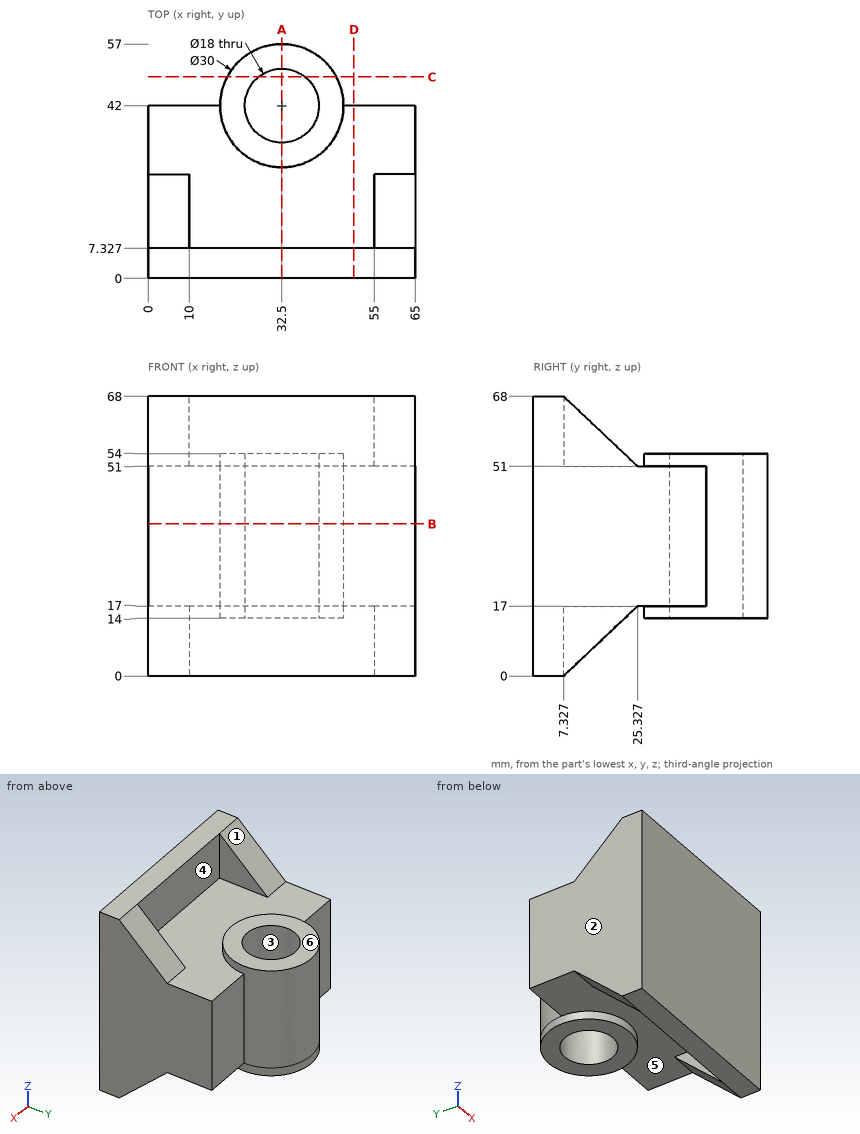
Job drawing, mm, ordinate dimensions from the low corner. One solid piece. A direction names the side the tool comes from. Round coordinates to 2 decimals unless told otherwise and drop trailing zeros. Order: outer loops, then holes, each group sorted by start corner. A loop starts at its lowest first (then second) coordinate and runs counter-clockwise, first axis right, second up. Notation, with made-up numbers: (79, 6) -> (98, 6) arc R21 cw to (98, 31) -> close; hole circle Ø9 at (23.5, 74.5). An arc over 180 degrees is marked (long way). Answer in a Markdown table with one row per item.
1) Mould opens along X. For the marked faces 1, 2 and 3 say: released by +X, released by -X, zero draft, split by the parting line, or undercut.
Values:
| item | result |
|---|---|
| face 1 | zero draft |
| face 2 | released by -X |
| face 3 | undercut |
2) Band-saw the part on B-B on z = 37. Give the cut face in (x, y), and give its area (3 significant figures).
Values:
| item | result |
|---|---|
| outline | (0, 0) -> (65, 0) -> (65, 42) -> (47.5, 42) arc R15 ccw to (17.5, 42) -> (0, 42) -> close; hole circle Ø18 at (32.5, 42) |
| area | 2,830 mm2 |
3) Wall check: L1, parallel to Y at x = 32, z = 28; L2, parallel to Y at x = 25, z = 53 (1 decimal); L3, parallel to Z at x = 13.5, y = 25. Give the ranges that are in metal, low to high.
Values:
| item | result |
|---|---|
| L1 | 0 to 33.01, 50.99 to 56.99 |
| L2 | 0 to 7.3, 29 to 37, 47 to 55 |
| L3 | 17 to 51 |
4) Pin check, flat tips, straight feed: P1, Ø13.5, axis at x = 33, z = 9.5, coming from the +Y side; P2, Ø14.5, axis at x = 32.5, y = 42, coming from the -Z side; P3, Ø19, axis at x = 52, z = 39.5, coming from the +Y side; P4, Ø19, axis at x = 9.5, z = 35.5, coming from the +Y side. Stop position of each tip, or through.
Values:
| item | result |
|---|---|
| P1 | y = 57 |
| P2 | through |
| P3 | y = 53.18 |
| P4 | y = 48.54 |
5) Which spindle directions (+Z, -Z, +X, -X, +Y, -Y) get a long thin tool onto all of the face, cutting with end or side? Do the marked faces 4, 5 and 6. Say none if no direction does.
Values:
| item | result |
|---|---|
| face 4 | +Z |
| face 5 | -Z |
| face 6 | +Z, +X, -X, +Y |
6) Band-saw the part on D-D on x = 50. Give the cut face in (y, z), and give its area (3 significant figures).
Values:
| item | result |
|---|---|
| outline | (0, 0) -> (7.33, 0) -> (7.33, 17) -> (42, 17) -> (42, 51) -> (7.33, 51) -> (7.33, 68) -> (0, 68) -> close |
| area | 1,680 mm2 |
7) Band-saw the part on A-A on x = 32.5. Give the cut face in (y, z).
Values:
| item | result |
|---|---|
| outline | (0, 0) -> (7.33, 0) -> (7.33, 17) -> (27, 17) -> (27, 14) -> (33, 14) -> (33, 54) -> (27, 54) -> (27, 51) -> (7.33, 51) -> (7.33, 68) -> (0, 68) -> close; (51, 14) -> (57, 14) -> (57, 54) -> (51, 54) -> close |
8) Band-saw the part on C-C on y = 49. Give the cut face in (x, z), and give its area (3 significant figures).
Values:
| item | result |
|---|---|
| outline | (19.23, 14) -> (26.84, 14) -> (26.84, 54) -> (19.23, 54) -> close; (38.16, 14) -> (45.77, 14) -> (45.77, 54) -> (38.16, 54) -> close |
| area | 609 mm2 |
